from build123d import *

# Parameters (mm, degrees)
F0_R           = 38.1
F0_R_2         = 12.7
F1_DEPTH       = 30
F2_SIZE        = 2
F4_D           = 7
F4_DEPTH       = 38.101
F5_D           = 7
F8_D           = 18
F8_DEPTH       = 10
F8_CBORE_D     = 25
F8_CBORE_DEPTH = 2
F8_TIP         = 5.4077455712
F9_SIZE        = 1


# Not quite as in the source:
# - a length typed as a fraction of an inch, garbled in the dataset ("3 / 203.2 mm" for 3/8 in), is restored


with BuildPart() as f1:
    # F0 (on Top) → F1 (new body)
    with BuildSketch(Plane.XY):
        Circle(F0_R)
        Circle(F0_R_2, mode=Mode.SUBTRACT)
    extrude(amount=F1_DEPTH)

    # F2
    f2_edges = [f1.edges().sort_by_distance(p)[0] for p in [
        (-38.1, 0, 30),
        (-38.1, 0, 0),
    ]]
    chamfer(f2_edges, length=F2_SIZE)

    # F4 (through all, one way)
    with BuildSketch(Plane(origin=(0, 0, 0), x_dir=(0, 1, 0), z_dir=(-1, 0, 0))):
        with Locations((0, -15)):
            Circle(F4_D / 2)
    extrude(amount=-F4_DEPTH, mode=Mode.SUBTRACT)

    # F5 (through all)
    with Locations(Plane.YZ):
        with Locations((0, 15)):
            Hole(F5_D / 2)

    # F8
    with Locations(Plane(origin=(-38.1, 0, 0), x_dir=(0, 1, 0), z_dir=(-1, 0, 0))):
        with Locations((0, -15.1190431789)):
            CounterBoreHole(F8_D / 2, F8_CBORE_D / 2, F8_CBORE_DEPTH, depth=F8_DEPTH)
            with Locations((0, 0, -(F8_DEPTH + F8_TIP / 2))):  # 118° drill point
                Cone(0, F8_D / 2, F8_TIP, mode=Mode.SUBTRACT)

    # F9
    f9_edges = [f1.edges().sort_by_distance(p)[0] for p in [
        (-12.7, 0, 0),
        (-12.7, 0, 30),
    ]]
    chamfer(f9_edges, length=F9_SIZE)


solid = f1.part
Design review of the part built by this model. Coordinates are the model's own, in mm. A direction names the side the tool comes from. Round coordinates to 2 decimals unless told otherwise and drop trailing zeros. Write each loop counter-clockwise with the first axis right and the second up, starting at its lowest first coordinate (ties: lowest second). Pieces come first, ordered by that corner, then holes. Notation, with made-up numbers: (73, 75) - (85, 75) arc R9 cw to (85, 80) - close; hole circle Ø2 at (30.25, 32.25). An arc over 180 degrees is marked (long way). Return JSON: item names as keys, results as strings. Group by question number.
Item 1: We need section B-B on x = 0. Write out the cut boundary in (y, z).
Item 2: Machinability: for faces 1 (the face through (12.114, 3.815, 14.804)), 2 (the face through (-32, 1.2, 6.2)), which of the approach directions +Z, -Z, +X, -X, +Y, -Y give a long, thin tool a straight path to every point of the face, cutting with its end or side? Answer none if there is none.
Item 3: The part is to be moulded in two halves that separate along Y. For faces 3 (the face through (-1, -16, 0)), 4 (the face through (-18.626, 0.759, 11.583)), 5 (the face through (36.34, 11.44, 14.82)), say which applies: pulls with the +Y half, pulls with the -Y half, needs draft (parallel to the pull), parting line crosses it, or undercut.
Item 4: Insertion check: P1, Ø1, axis at y = 13, z = 23, coming from the -X side; P2, Ø4, axis at y = -8, z = 23.5, coming from the -X side; P3, Ø8, axis at x = 9.5, z = 9.5, coming from the +Y side; P4, Ø6.5, axis at y = 0, z = 15, coming from the -X side. Each pin has a flat end and moves straight along its axis. Give the tip position at first contact, or say it passes through.
Item 5: We need section A-A on y = 0. Give the number of separate pieces and of enclosed holes in the cut face, and give its area (3 significant figures).
Item 6: For probe 1 along X at (y, z) = (8, 7.75); probe 2 along Y at (x, z) = (0, 22.25); probe 3 along Y at (x, z) = (-4.5, 26.5), list the stretches that pass through material, from the lowest coordinate up. Write a range as [from, to].
Item 7: We need section C-C on z = 25.5. Write out the cut boundary in (x, y).
Model answer:
{
 "1": {"outline": "(-38.1, 2) - (-36.1, 0) - (-13.7, 0) - (-12.7, 1) - (-12.7, 29) - (-13.7, 30) - (-36.1, 30) - (-38.1, 28) - close; (12.7, 1) - (13.7, 0) - (36.1, 0) - (38.1, 2) - (38.1, 28) - (36.1, 30) - (13.7, 30) - (12.7, 29) - close"},
 "2": {"face 1": "+Z, -Z", "face 2": "-X"},
 "3": {"face 3": "needs draft", "face 4": "undercut", "face 5": "parting line crosses it"},
 "4": {"P1": "stops at x = -35.99", "P2": "stops at x = -37.41", "P3": "stops at y = 37.7", "P4": "passes through"},
 "5": {"separate pieces": "4", "enclosed holes": "0", "area": "1,020 mm²"},
 "6": {"probe 1": "x = [-36.1, -9.86], [9.86, 37.25]", "probe 2": "y = [-38.1, -12.7], [12.7, 38.1]", "probe 3": "y = [-37.83, -11.88], [11.88, 37.83]"},
 "7": {"outline": "(-37.46, -6.96) arc R38.1 ccw (long way) to (-37.46, 6.96) - (-36.1, 6.96) - (-36.1, -6.96) - close; hole circle Ø25.4 at (0, 0)"}
}
